Verification items for the finished model (mm, model axes). A direction names the side the tool comes from. Round coordinates to 2 decimals unless told otherwise and drop trailing zeros. Order: outer loops, then holes, each group sorted by start corner. A loop starts at its lowest first (then second) coordinate and runs counter-clockwise, first axis right, second up. Notation, with made-up numbers: M 31.5,34.25 L 35.5,34.25 A23 ccw 35.5,58.25 Z; hole C 28,48.5 d9. An arc over 180 degrees is marked long. Return JSON: item names as keys, results as strings. Group by question number.
from build123d import *

# Parameters (mm, degrees)
F0_W          = 50.8
F0_H          = 50.8
F1_DEPTH      = 50.8
F2_R          = 20.32
F4_DEPTH      = 28.575
F4_DEPTH_BACK = 28.575
F5_T1_DEPTH   = 171.45
F5_T3_DEPTH   = 173.3631305569


# Not quite as in the source:
# - a fillet or chamfer that OpenCascade refuses, or shapes differently, is made with other operations: its cross-section is extruded or revolved along the edge and cut away or added


with BuildPart() as f1:
    # F0 (on Top) → F1 (new body)
    with BuildSketch(Plane.XY):
        Rectangle(F0_W, F0_H)
    extrude(amount=F1_DEPTH)

    # F2
    f2_edges = [f1.edges().sort_by_distance(p)[0] for p in [
        (0, 25.4, 50.8),
        (-25.4, 0, 50.8),
        (0, -25.4, 50.8),
        (25.4, 0, 50.8),
        (-25.4, 25.4, 25.4),
        (-25.4, -25.4, 25.4),
        (-25.4, 0, 0),
        (25.4, -25.4, 25.4),
        (0, -25.4, 0),
        (25.4, 25.4, 25.4),
        (25.4, 0, 0),
        (0, 25.4, 0),
    ]]
    fillet(f2_edges, radius=F2_R)

    # F3 (on Right) → F4 (join, two sides)
    with BuildSketch(Plane.YZ) as f4_sk:
        with BuildLine():
            Line((0, 23.585671559), (0, 30.6485332549))
            add(Edge.make_bspline(
                [(0, 30.6485332549), (0, 33.0861583352), (7.1330016043, 33.8045146668), (15.9690734978, 28.3277997784), (21.6986452978, 15.0790064451), (22.6556025445, 8.0415420234)],
                knots=[0, 0, 0, 0, 0.2426532196, 0.5552693869, 1, 1, 1, 1], degree=3))
            add(Edge.make_bspline(
                [(22.6556025445, 8.0415420234), (25.1164599813, 8.5749836186), (27.5161694097, 10.7134623968), (29.5368228108, 15.9953534603), (29.541708529, 20.0420022011)],
                knots=[0, 0, 0, 0, 0.4304337748, 1, 1, 1, 1], degree=3))
            Line((29.541708529, 20.0420022011), (29.541708529, 52.6639260352))
            Line((29.541708529, 52.6639260352), (-29.5214220279, 52.6639260352))
            Line((-29.5214220279, 52.6639260352), (-5.094319582, 30.5475965142))
            Line((-5.094319582, 30.5475965142), (-5.094319582, 23.585671559))
            Line((-5.094319582, 23.585671559), (0, 23.585671559))
        make_face()
    extrude(amount=F4_DEPTH)
    extrude(f4_sk.sketch, amount=-F4_DEPTH_BACK)

    # F5: fillet of radius 22.86 on 3 edges, made by hand

    # F5_s2 → F5_t1 (cut)
    with BuildSketch(Plane.YZ.offset(-85.725)):
        with BuildLine():
            ThreePointArc((29.541708529, 29.8039260352), (22.8461695469, 45.9683870531), (6.681708529, 52.6639260352))
            Line((6.681708529, 52.6639260352), (29.541708529, 52.6639260352))
            Line((29.541708529, 52.6639260352), (29.541708529, 29.8039260352))
        make_face()
    extrude(amount=F5_T1_DEPTH, mode=Mode.SUBTRACT)

    # F5_s4 → F5_t3 (cut)
    with BuildSketch(Plane.XZ.offset(-86.691708529)):
        with BuildLine():
            ThreePointArc((-28.575, 29.8039260352), (-21.8794610179, 45.9683870531), (-5.715, 52.6639260352))
            Line((-5.715, 52.6639260352), (-28.575, 52.6639260352))
            Line((-28.575, 52.6639260352), (-28.575, 29.8039260352))
        make_face()
        with BuildLine():
            ThreePointArc((28.575, 29.8039260352), (21.8794610179, 45.9683870531), (5.715, 52.6639260352))
            Line((5.715, 52.6639260352), (28.575, 52.6639260352))
            Line((28.575, 52.6639260352), (28.575, 29.8039260352))
        make_face()
    extrude(amount=F5_T3_DEPTH, mode=Mode.SUBTRACT)


solid = f1.part
1. Draft check along Y on faces 1 (the face through (0.4, -22.91, 46.68)), 2 (the face through (-24.57, 10.83, 24.34)), 3 (the face through (-25.4, 1, 24)), 4 (the face through (0, -11, 52.664)). Enter one of: +Y half, -Y half, draft (parallel to the pull), parting line (faces both ways), or undercut.
2. Cross-section at A-A (y = -15.5). Enter the section's corners in (x, z) (3 decimals).
3. Go/stop test with flat-tipped pins: pin 1 (1.6 mm diameter, centred on x = 27.5, y = -2.5, fed in from -Z); pin 2 (2 mm diameter, centred on x = 15, z = 35, fed in from +Y); pin 3 (3 mm diameter, centred on y = 0.5, z = 27.5, fed in from -X) (3 decimals); pin 4 (3 mm diameter, centred on y = -6, z = 40, fed in from +X). Record where each tip stops, or that it passes through.
4. Access from +Z, -Z, +X, -X, +Y, -Y to the whole of each face (thin tool, end or side, straight path). Record for faces 5 (the face through (-27, 0, 27)), 6 (the face through (27, 0, 27)), 7 (the face through (-27, -3, 23.586)), 8 (the face through (27, -5.094, 27)).
5. Cross-section at B-B (z = 48.5). Enter the section's corners in (x, y), plus the area to 3 significant figures.
6. Thickness scan on line 1 along X through (y, z) = (3, 41.5); line 2 along Z through (x, y) = (-15, -15); line 3 along Y through (x, z) = (3, 13). Record the ranges inside material, lowest first. Write a range as from..to.
Computed:
{
 "1": {"face 1": "-Y half", "face 2": "undercut", "face 3": "undercut", "face 4": "draft"},
 "2": {"outline": "M -26.191,39.969 L -19.719,39.969 A17.445 ccw -22.525,30.48 L -22.525,20.32 A17.445 ccw -5.08,2.875 L 5.08,2.875 A17.445 ccw 22.525,20.32 L 22.525,30.48 A17.445 ccw 19.719,39.969 L 26.191,39.969 A22.86 ccw 5.715,52.664 L -5.715,52.664 A22.86 ccw Z"},
 "3": {"pin 1": "stops at z = 23.59", "pin 2": "stops at y = 29.15", "pin 3": "stops at x = -28.575", "pin 4": "stops at x = 26.86"},
 "4": {"face 5": "-Z, -X", "face 6": "-Z, +X", "face 7": "-Z, -X, -Y", "face 8": "-Z, +X, -Y"},
 "5": {"outline": "M -18.87,-24.92 L 18.87,-24.92 L 18.87,19.84 L -18.87,19.84 Z", "area": "1,690 mm²"},
 "6": {"line 1": "x = -25.36..25.36", "line 2": "z = 5.62..50.69", "line 3": "y = -24.04..28.17"}
}
